Build history of the part. All positions in model axes, mm. Give positions to 0.01 mm unless a question says otherwise; leave off trailing zeros. Loops run counter-clockwise (first coordinate to the right, second up) from the corner with the lowest first, then second, coordinate; pieces in that order, holes last. Notation, with made-up numbers: M 51,70.5 L 80,70.5 A11 ccw 80,82.5 Z; hole C 27.25,-26 d1. An arc over 180 degrees is marked long. Answer as a JSON object with one key per item and string values. Group by question number.
1. Drop a flat-ended pin along its axis: pin 1 Ø3 at (x, y) = (-2, 3) entering from +Z. Give the stop position or say it passes through.
2. Drill centre lines: line 1 along Z through (x, y) = (0, 0); line 2 along Z through (x, y) = (-2.5, 1.25). Where is each one in solid material? Low to high. Write a range as [from, to].
3. Slice it at A-A (x = 0). List the corners of the cut face in (y, z).
4. Slice it at C-C (y = -3.25). List the corners of the cut face in (x, z), then the cut area to 3 significant figures.
5. Mould opens along X. For faces 1 (the face through (13, -4, 9)), 2 (the face through (12.932, -0.053, 5.362)), 3 (the face through (-4.336, 0.053, 19.524)) say: released by +X, released by -X, zero draft, split by the parting line, or undercut.
6. Slice it at B-B (z = 0). List the corners of the cut face in (x, y), then the cut area to 3 significant figures.
from build123d import *

# Parameters (mm, degrees)
SKETCH1_R           = 20
SKETCH1_R_2         = 14
BOSS_EXTRUDE1_DEPTH = 4
CHAMFER1_SIZE       = 0.2


with BuildPart() as part:
    # Sketch1 → Boss-Extrude1 (new body, symmetric)
    with BuildSketch(Plane(origin=(0, 0, 0), x_dir=(1, 0, 0), z_dir=(0, 1, 0))):
        Circle(SKETCH1_R)
        Circle(SKETCH1_R_2, mode=Mode.SUBTRACT)
    extrude(amount=BOSS_EXTRUDE1_DEPTH, both=True)

    # Chamfer1
    chamfer1_edges = [part.edges().sort_by_distance(p)[0] for p in [
        (-20, -4, 0),
        (-20, 4, 0),
        (-14, -4, 0),
        (-14, 4, 0),
    ]]
    chamfer(chamfer1_edges, length=CHAMFER1_SIZE)


solid = part.part
Established:
{
 "1": {"pin 1": "stops at z = 19.99"},
 "2": {"line 1": "z = [-20, -14], [14, 20]", "line 2": "z = [-19.84, -13.77], [13.77, 19.84]"},
 "3": {"outline": "M -4,-19.8 L -3.8,-20 L 3.8,-20 L 4,-19.8 L 4,-14.2 L 3.8,-14 L -3.8,-14 L -4,-14.2 Z; M -4,14.2 L -3.8,14 L 3.8,14 L 4,14.2 L 4,19.8 L 3.8,20 L -3.8,20 L -4,19.8 Z"},
 "4": {"outline": "C 0,0 d40; hole C 0,0 d28", "area": "641 mm^2"},
 "5": {"face 1": "zero draft", "face 2": "undercut", "face 3": "split by the parting line"},
 "6": {"outline": "M -20,-3.8 L -19.8,-4 L -14.2,-4 L -14,-3.8 L -14,3.8 L -14.2,4 L -19.8,4 L -20,3.8 Z; M 14,-3.8 L 14.2,-4 L 19.8,-4 L 20,-3.8 L 20,3.8 L 19.8,4 L 14.2,4 L 14,3.8 Z", "area": "95.8 mm^2"}
}
